```python
from build123d import *

# Parameters (mm, degrees)
SKETCH1_W           = 68
SKETCH1_H           = 29.5
BOSS_EXTRUDE1_DEPTH = 2.5
BOSS_EXTRUDE2_DEPTH = 30
CUT_EXTRUDE1_DEPTH  = 50.5
FILLET1_R           = 1.5
FILLET2_R           = 1


with BuildPart() as part:
    # Sketch1 → Boss-Extrude1 (new body)
    with BuildSketch(Plane(origin=(0, 0, 0), x_dir=(1, 0, 0), z_dir=(0, 1, 0))):
        Rectangle(SKETCH1_W, SKETCH1_H)
    extrude(amount=BOSS_EXTRUDE1_DEPTH)

    # Sketch2 → Boss-Extrude2 (add)
    with BuildSketch(Plane(origin=(0, 2.5, 0), x_dir=(1, 0, 0), z_dir=(0, 1, 0))):
        Polygon((-31.5, -6.75), (-34, -6.75), (-34, -14.75), (0, -14.75), (0, -12.25), (-31.5, -12.25), align=None)
        Polygon((0, -12.25), (0, -14.75), (34, -14.75), (34, -6.75), (31.5, -6.75), (31.5, -12.25), align=None)
        Polygon((34, 14.75), (0, 14.75), (0, 12.25), (31.5, 12.25), (31.5, 6.75), (34, 6.75), align=None)
        Polygon((0, 14.75), (-34, 14.75), (-34, 6.75), (-31.5, 6.75), (-31.5, 12.25), (0, 12.25), align=None)
    extrude(amount=BOSS_EXTRUDE2_DEPTH)

    # Sketch3 → Cut-Extrude1 (cut)
    with BuildSketch(Plane.XY.offset(-12.25)):
        Polygon((7, 19.5), (7, 28.5), (0, 28.5), (-7, 28.5), (-7, 19.5), align=None)
    extrude(amount=CUT_EXTRUDE1_DEPTH, mode=Mode.SUBTRACT)

    # Fillet1
    fillet1_edges = [part.edges().sort_by_distance(p)[0] for p in [
        (0, 0, 14.75),
        (-34, 0, 0),
        (-34, 16.25, -14.75),
        (34, 16.25, -14.75),
        (34, 16.25, 14.75),
        (-34, 16.25, 14.75),
        (31.5, 17.5, 12.25),
        (-31.5, 17.5, 12.25),
        (-31.5, 17.5, -12.25),
        (31.5, 17.5, -12.25),
        (7, 24, 12.25),
        (0, 28.5, 12.25),
        (-7, 24, 12.25),
        (0, 19.5, 12.25),
        (0, 0, -14.75),
        (34, 0, 0),
    ]]
    fillet(fillet1_edges, radius=FILLET1_R)

    # Fillet2
    fillet2_edges = [part.edges().sort_by_distance(p)[0] for p in [
        (-34, 17.5, 6.75),
        (34, 17.5, 6.75),
        (34, 17.5, -6.75),
        (-34, 17.5, -6.75),
    ]]
    fillet(fillet2_edges, radius=FILLET2_R)


solid = part.part
```
Here's how the part is built. I have some questions about the finished solid (model axes, mm). A direction names the side the tool comes from. Coordinates: 2 decimals unless noted, no trailing zeros. Loops run counter-clockwise (first coordinate to the right, second up) from the corner with the lowest first, then second, coordinate; pieces in that order, holes last. Notation, with made-up numbers: (88.25, 11) -> (98.25, 11) arc R7 ccw to (98.25, 23) -> close; hole circle Ø6 at (15.5, 35). An arc over 180 degrees is marked (long way). Return JSON: item names as keys, results as strings.
1) If we section it at C-C, the plane x = 6: Write out the boundary of the cut face in (y, z).
Results below:
{"outline": "(0, -13.25) arc R1.5 ccw to (1.5, -14.75) -> (32.5, -14.75) -> (32.5, -12.25) -> (2.5, -12.25) -> (2.5, 12.25) -> (18, 12.25) arc R1.5 ccw to (19.5, 13.75) -> (19.5, 14.75) -> (1.5, 14.75) arc R1.5 ccw to (0, 13.25) -> close; (28.5, 13.75) arc R1.5 ccw to (30, 12.25) -> (32.5, 12.25) -> (32.5, 14.75) -> (28.5, 14.75) -> close"}
2) If we section it at D-D, the plane z = -9.75: Write out the boundary of the cut face in (x, y).
Results below:
{"outline": "(-34, 1.5) arc R1.5 ccw to (-32.5, 0) -> (32.5, 0) arc R1.5 ccw to (34, 1.5) -> (34, 32.5) -> (31.5, 32.5) -> (31.5, 2.5) -> (-31.5, 2.5) -> (-31.5, 32.5) -> (-34, 32.5) -> close"}
3) For faces 1 (the face through (0.45, 0.43, -14.3)), 2 (the face through (-32, 17, -6.75)), 3 (the face through (31.5, 17, -9)), 4 (the face through (-34, 17, -9)), 5 (the face through (0.12, 28.95, 12.68)), which set-ups out of +Z, -Z, +X, -X, +Y, -Y let a thin tool reach every point of the face, with its end or its side?
Results below:
{"face 1": "-Z, +X, -X, -Y", "face 2": "+X, -X, +Y", "face 3": "+Y", "face 4": "+Z, -Z, -X, +Y, -Y", "face 5": "none"}
4) I need wall thicknesses on line 1 (Z direction, x = 28.5, y = 29); line 2 (Y direction, x = 23.5, z = 4.25); line 3 (Z direction, x = -31, y = 15.5). Which ranges of each line are inside material? Lowest first, please. Write a range as from..to.
Results below:
{"line 1": "-14.75..-12.25, 12.25..14.75", "line 2": "0..2.5", "line 3": "-14.75..-11.87, 11.87..14.75"}
5) If we section it at B-B, the plane y = 26.5: Count the separate pieces of the cut face and the enclosed holes in it, then the cut area to 3 significant figures.
Results below:
{"separate pieces": "3", "enclosed holes": "0", "area": "358 mm²"}
6) Thinking about a two-plate mould opening in X: for faces 6 (the face through (0, 32.5, 13)), 7 (the face through (31.05, 17.71, 11.82)), 8 (the face through (-33.57, 16.78, -14.3)), 9 (the face through (31.05, 17.71, -11.82)), which applies, +X half, -X half, draft (parallel to the pull), parting line (faces both ways), or undercut?
Results below:
{"face 6": "draft", "face 7": "undercut", "face 8": "-X half", "face 9": "undercut"}
7) If we section it at A-A, the plane y = 5.5: Write out the boundary of the cut face in (x, z), then the cut area to 3 significant figures.
Results below:
{"outline": "(-34, -13.25) arc R1.5 ccw to (-32.5, -14.75) -> (32.5, -14.75) arc R1.5 ccw to (34, -13.25) -> (34, -7.75) arc R1 ccw to (33, -6.75) -> (31.5, -6.75) -> (31.5, -10.75) arc R1.5 cw to (30, -12.25) -> (-30, -12.25) arc R1.5 cw to (-31.5, -10.75) -> (-31.5, -6.75) -> (-33, -6.75) arc R1 ccw to (-34, -7.75) -> close; (-34, 7.75) arc R1 ccw to (-33, 6.75) -> (-31.5, 6.75) -> (-31.5, 10.75) arc R1.5 cw to (-30, 12.25) -> (30, 12.25) arc R1.5 cw to (31.5, 10.75) -> (31.5, 6.75) -> (33, 6.75) arc R1 ccw to (34, 7.75) -> (34, 13.25) arc R1.5 ccw to (32.5, 14.75) -> (-32.5, 14.75) arc R1.5 ccw to (-34, 13.25) -> close", "area": "394 mm²"}
8) Will these pins go through, and if not, where does the flat tip stop? pin 1 (0.8 mm diameter, centred on x = 3, z = 14, fed in from -Y); pin 2 (12 mm diameter, centred on x = 6.5, z = -0.5, fed in from +Y); pin 3 (1.1 mm diameter, centred on y = 24, z = 14.5, fed in from -X); pin 4 (2 mm diameter, centred on y = 21.5, z = -5, fed in from +X).
Results below:
{"pin 1": "y = 0.04", "pin 2": "y = 2.5", "pin 3": "x = -33.83", "pin 4": "through"}
